Autodesk Inventor part; units mm, degrees
ref_plane "YZ Plane" through (0, 0, 0) normal (1, 0, 0) x (0, 1, 0)
ref_plane "XZ Plane" through (0, 0, 0) normal (0, 1, 0) x (-1, 0, 0)
ref_plane "XY Plane" through (0, 0, 0) normal (0, 0, 1) x (1, 0, 0)
sketch "Sketch1" plane through (0, 0, 0) normal (0, 0, 1) x (1, 0, 0)
  circle A0 centre (0, 0) radius 56.5
  dimension "d0" = 113
extrude "Extrusion1" add sketch "Sketch1" along normal blind 20
thread "Thread1"
chamfer "Chamfer1" distance 5 angle 45 2 edges at (-56.5, 0, 20) (-56.5, 0, 0)
sketch "Sketch2" plane through (0, 0, 20) normal (0, 0, 1) x (1, 0, 0)
  point P0 (0, 0)
  point P1 (0.2077, 1.3498)
hole "Hole1" at (0.2077, 1.3498, 20) direction (0, 0, -1) diameter 15 depth 20 tip angle 118
properties part number "new_encoder"
Check sheet for the modelled part. Datum: model origin and axes. Units: mm. Give positions to 0.01 mm unless a question says otherwise; leave off trailing zeros. Write each loop counter-clockwise with the first axis right and the second up, starting at its lowest first coordinate (ties: lowest second). Pieces come first, ordered by that corner, then holes.
Item 1: Cross-section at B-B (z = 7.75). Enter the section's corners in (x, y).
Item 2: Gauge pin test, flat ends, axial feed: pin 1 (10 mm diameter, centred on y = -0.5, z = 3.5, fed in from -X); pin 2 (3 mm diameter, centred on x = 8.5, z = 9.5, fed in from -Y); pin 3 (8 mm diameter, centred on x = 10, z = 7.5, fed in from +Y); pin 4 (1 mm diameter, centred on y = -21, z = 15.5, fed in from +X). Record the tip position at first contact, or that the pin passes through.
Item 3: Scan lines: L1, parallel to X at y = -2.5, z = 5.25; L2, parallel to Y at x = -0.5, z = 16.75; L3, parallel to X at y = 5.5, z = 4.5. Record each from-to range of solid material in increasing order.
Item 4: Draft check along Y on faces 1 (the face through (-4.86, 6.88, 9.86)), 2 (the face through (-38.188, -35.018, 19.687)), 3 (the face through (-1, -11, 0)). Enter one of: released by +Y, released by -Y, zero draft, split by the parting line, or undercut.
Item 5: Cross-section at A-A (y = 0). Enter the section's corners in (x, z), and give its area (3 significant figures).
Report:
1. outline: circle Ø113 at (0, 0); hole circle Ø15 at (0.21, 1.35)
2. pin 1: stops at x = -56.5
2. pin 2: stops at y = -56.06
2. pin 3: stops at y = 56.18
2. pin 4: stops at x = 52.49
3. L1: x = -56.44 to -6.23, 6.64 to 56.44
3. L2: y = -54.75 to -6.12, 8.82 to 54.75
3. L3: x = -55.73 to -6.04, 6.45 to 55.73
4. face 1: undercut
4. face 2: split by the parting line
4. face 3: zero draft
5. outline: (-56.5, 5) - (-51.5, 0) - (-7.17, 0) - (-7.17, 20) - (-51.5, 20) - (-56.5, 15) - close; (7.59, 0) - (51.5, 0) - (56.5, 5) - (56.5, 15) - (51.5, 20) - (7.59, 20) - close
5. area: 1,910 mm2
